from build123d import *

# Parameters (mm, degrees)
EXTRUDE1_DEPTH    = 5.85
EXTRUDE2_START    = 9.05
SKETCH2_R         = 2.25
EXTRUDE2_DEPTH    = 2.1
EXTRUDE3_START    = 12.95
EXTRUDE3_DEPTH    = 3.2
EXTRUDE6_START    = 16.15
SKETCH6_R         = 1.25
EXTRUDE6_DEPTH    = 1
EXTRUDE4_START    = 16.15
SKETCH4_R         = 2.85
SKETCH4_R_2       = 1.5
EXTRUDE4_DEPTH    = 4
EXTRUDE5_START    = 16.15
EXTRUDE5_DEPTH    = 4
CIRPATTERN1_COUNT = 24
FILLET1_R         = 1
FILLET2_R         = 0.5


with BuildPart() as part:
    # Sketch1 → Extrude1 (new, symmetric)
    with BuildSketch(Plane.XY):
        Polygon((-14.9, -12.95), (-14.9, 6.95), (-19.9, 6.95), (-19.9, 9.05), (-14.9, 9.05), (-14.9, 12.95), (14.9, 12.95), (14.9, 9.05), (19.9, 9.05), (19.9, 6.95), (14.9, 6.95), (14.9, -12.95), align=None)
    extrude(amount=EXTRUDE1_DEPTH, both=True)

    # Sketch2 → Extrude2 (cut)
    with BuildSketch(Plane(origin=(0, 0, 0), x_dir=(1, 0, 0), z_dir=(0, 1, 0)).offset(EXTRUDE2_START)):
        with Locations((-18.1, 0)):
            Circle(SKETCH2_R)
        with Locations((18.1, 0)):
            Circle(SKETCH2_R)
    extrude(amount=-EXTRUDE2_DEPTH, mode=Mode.SUBTRACT)

    # Sketch3 → Extrude3 (add)
    with BuildSketch(Plane(origin=(0, 0, 0), x_dir=(1, 0, 0), z_dir=(0, 1, 0)).offset(EXTRUDE3_START)):
        with BuildLine():
            Line((7.846183973, 5.85), (1.953816027, 5.85))
            ThreePointArc((1.953816027, 5.85), (0.884733475, 5.174952631), (-0.034732824, 4.307076961))
            ThreePointArc((-0.034732824, 4.307076961), (-6.25, 0), (-0.034732824, -4.307076961))
            ThreePointArc((-0.034732824, -4.307076961), (0.884733475, -5.174952631), (1.953816027, -5.85))
            Line((1.953816027, -5.85), (7.846183973, -5.85))
            ThreePointArc((7.846183973, -5.85), (11.45, 0), (7.846183973, 5.85))
        make_face()
    extrude(amount=EXTRUDE3_DEPTH)

    # Sketch6 → Extrude6 (add)
    with BuildSketch(Plane(origin=(0, 0, 0), x_dir=(1, 0, 0), z_dir=(0, 1, 0)).offset(EXTRUDE6_START)):
        with Locations((-1.65, 0)):
            Circle(SKETCH6_R)
    extrude(amount=EXTRUDE6_DEPTH)

    # Sketch4 → Extrude4 (add)
    with BuildSketch(Plane(origin=(0, 0, 0), x_dir=(1, 0, 0), z_dir=(0, 1, 0)).offset(EXTRUDE4_START)):
        with Locations((4.9, 0)):
            Circle(SKETCH4_R)
        with Locations((4.9, 0)):
            Circle(SKETCH4_R_2, mode=Mode.SUBTRACT)
    extrude(amount=EXTRUDE4_DEPTH)

    # Sketch5 → Extrude5 (cut)
    with BuildSketch(Plane(origin=(0, 0, 0), x_dir=(1, 0, 0), z_dir=(0, 1, 0)).offset(EXTRUDE5_START)):
        with BuildLine():
            Line((4.005073985, -2.705846897), (4.447115963, -2.373874784))
            Line((4.447115963, -2.373874784), (4.735892559, -2.845271296))
            ThreePointArc((4.735892559, -2.845271296), (4.365914093, -2.799509286), (4.005073985, -2.705846897))
        make_face()
    extrude5 = extrude(amount=EXTRUDE5_DEPTH, mode=Mode.SUBTRACT)

    # CirPattern1: Extrude5 ×24 about axis
    cirpattern1_axis = Axis((4.9, 0, 0), (0, 1, 0))
    for i in range(1, CIRPATTERN1_COUNT):
        add(extrude5.rotate(cirpattern1_axis, i * 360 / CIRPATTERN1_COUNT), mode=Mode.SUBTRACT)

    # Fillet1
    fillet1_edges = [part.edges().sort_by_distance(p)[0] for p in [
        (11.373091986, 12.95, -5.85),
        (14.9, 12.95, 0),
        (11.373091986, 12.95, 5.85),
        (-6.473091986, 12.95, -5.85),
        (-14.9, 12.95, 0),
        (-6.473091986, 12.95, 5.85),
        (14.9, -12.95, 0),
        (-14.9, -12.95, 0),
        (0, -12.95, 5.85),
        (0, -12.95, -5.85),
        (14.9, 11, -5.85),
        (-14.9, 11, -5.85),
        (-14.9, 11, 5.85),
        (14.9, 11, 5.85),
        (14.9, -3, 5.85),
        (14.9, -3, -5.85),
        (-14.9, -3, -5.85),
        (-14.9, -3, 5.85),
    ]]
    fillet(fillet1_edges, radius=FILLET1_R)

    # Fillet2
    fillet2_edges = [part.edges().sort_by_distance(p)[0] for p in [
        (-2.9, 17.15, 0),
        (-2.9, 16.15, 0),
    ]]
    fillet(fillet2_edges, radius=FILLET2_R - 0.0001)  # a hair under: the kernel refuses the full size


solid = part.part
Here's how the part is built. I have some questions about the finished solid (model axes, mm). A direction names the side the tool comes from. Coordinates: 2 decimals unless noted, no trailing zeros. Loops run counter-clockwise (first coordinate to the right, second up) from the corner with the lowest first, then second, coordinate; pieces in that order, holes last.
1. I need wall thicknesses on L1, parallel to Z at x = -18, y = 7; L2, parallel to Y at x = -7.5, z = 3; L3, parallel to X at y = -8, z = 3.25. Which ranges of each line are inside material? Lowest first, please.
2. For faces 1 (the flat face through (-14.9, -3, 0)), 2 (the flat face through (-14.9, 10, 0)), 3 (the cylindrical face through (10.915, 12.649, -5.565)), 4 (the cylindrical face through (14.599, -2.632, -5.565)), which set-ups out of +Z, -Z, +X, -X, +Y, -Y let a thin tool reach every point of the face, with its end or its side?
3. For P1, Ø5, axis at y = -0.5, z = -1, coming from the +X side; P2, Ø3, axis at y = 10, z = -1.5, coming from the +X side; P3, Ø1.4, axis at x = 12.5, z = 0.5, coming from the +Y side; P4, Ø1.8, axis at x = 4.9, z = 0, coming from the +Y side, each with a flat end and sliding along its axis, tell me the tip position at first contact or that it passes through.
4. Imagine slicing it at C-C, the plane x = -12. Please give me the cut outline in (y, z), and give its area (3 significant figures).
5. Imagine slicing it at D-D, the plane y = 13.5. Please give me the cut outline in (x, z), and give its area (3 significant figures).
6. If we mould it in two halves opening along X, with no side actions, what happens to faces 5 (the flat face through (19.9, 8, 4)), 6 (the cylindrical face through (-0.195, -12.665, -5.549)), 7 (the cylindrical face through (6.286, 18.122, 0.575)), 8 (the flat face through (5, 16.15, 0))? For each: pulls with the +X half, pulls with the -X half, needs draft (parallel to the pull), parting line crosses it, or undercut.
7. Imagine slicing it at A-A, the plane x = -18.1. Please give me the cut outline in (y, z).
8. Imagine slicing it at B-B, the plane y = 10. Please give me the cut outline in (x, z).
Taken from the geometry:
1. L1: z = -5.85 to -2.25, 2.25 to 5.85
1. L2: y = -12.95 to 12.95
1. L3: x = -14.9 to 14.9
2. face 1: +Z, -Z, -X, -Y
2. face 2: +Z, -Z, -X, +Y
2. face 3: -Z, +X, +Y
2. face 4: -Z, +X, -Y
3. P1: stops at x = 14.9
3. P2: stops at x = 19.9
3. P3: stops at y = 12.95
3. P4: stops at y = 16.15
4. outline: (-12.95, -4.85) arc R1 ccw to (-11.95, -5.85) - (11.95, -5.85) arc R1 ccw to (12.95, -4.85) - (12.95, 4.85) arc R1 ccw to (11.95, 5.85) - (-11.95, 5.85) arc R1 ccw to (-12.95, 4.85) - close
4. area: 302 mm2
5. outline: (-0.03, -4.31) arc R6.55 ccw to (1.95, -5.85) - (7.85, -5.85) arc R6.55 ccw to (7.85, 5.85) - (1.95, 5.85) arc R6.55 ccw to (-0.03, 4.31) arc R4.6 ccw (long way) to start
5. area: 167 mm2
6. face 5: pulls with the +X half
6. face 6: needs draft
6. face 7: undercut
6. face 8: undercut
7. outline: (6.95, -5.85) - (9.05, -5.85) - (9.05, -2.25) - (6.95, -2.25) - close; (6.95, 2.25) - (9.05, 2.25) - (9.05, 5.85) - (6.95, 5.85) - close
8. outline: (-14.9, -4.85) arc R1 ccw to (-13.9, -5.85) - (13.9, -5.85) arc R1 ccw to (14.9, -4.85) - (14.9, 4.85) arc R1 ccw to (13.9, 5.85) - (-13.9, 5.85) arc R1 ccw to (-14.9, 4.85) - close
